Design review of the part built by this model. Coordinates are the model's own, in mm. A direction names the side the tool comes from. Coordinates: 2 decimals unless noted, no trailing zeros. Order: outer loops, then holes, each group sorted by start corner. A loop starts at its lowest first (then second) coordinate and runs counter-clockwise, first axis right, second up. Notation, with made-up numbers: M -24.75,9 L 13.25,9 A25 cw 13.25,41 Z; hole C 20,12.5 d3. An arc over 180 degrees is marked long. Answer in a Markdown table with one row per item.
Autodesk Inventor part; units mm, degrees
ref_plane "YZ Plane" through (0, 0, 0) normal (1, 0, 0) x (0, 1, 0)
ref_plane "XZ Plane" through (0, 0, 0) normal (0, 1, 0) x (-1, 0, 0)
ref_plane "XY Plane" through (0, 0, 0) normal (0, 0, 1) x (1, 0, 0)
sketch "Boceto16" plane through (0, 0, 0) normal (0, 0, 1) x (1, 0, 0)
  line L0 (-21.15, 21.15) -> (21.15, 21.15)
  line L1 (21.15, 21.15) -> (21.15, -21.15)
  line L2 (21.15, -21.15) -> (-21.15, -21.15)
  line L3 (-21.15, -21.15) -> (-21.15, 21.15)
  line L4 (2.3235, 0) -> (0, 0)
  line L5 (0, 0) -> (0, 2.4447)
  dimension "d75" = 42.3
  dimension "d76" = 42.3
extrude "Extrusión15" add sketch "Boceto16" along normal blind 15
sketch "Boceto17" plane through (0, 0, 15) normal (0, 0, 1) x (1, 0, 0)
  circle A0 centre (15.5, 15.5) radius 1.5
  point P0 (0, 0)
  dimension "d79" = 3
  dimension "d80" = 15.5
  dimension "d81" = 15.5
extrude "Extrusión16" cut sketch "Boceto17" against normal through all
pattern_linear "Patrón rectangular2" count 2 spacing 31 along (-1, 0, 0) count 2 spacing 31 along (0, -1, 0) of "Extrusión16"
sketch "Boceto18" plane through (0, 0, 15) normal (0, 0, 1) x (1, 0, 0)
  line L0 (-21.15, -21.15) -> (21.15, -21.15)
  line L1 (-21.15, 21.15) -> (-21.15, -21.15)
  line L2 (21.15, -21.15) -> (-21.15, -21.15)
  line L3 (-21.15, -21.15) -> (-21.15, 11.85)
  line L4 (-21.15, 11.85) -> (21.15, 11.85)
  line L5 (21.15, 11.85) -> (21.15, -21.15)
  circle A0 centre (-15.5, -15.5) radius 1.5
  circle A1 centre (15.5, -15.5) radius 1.5
  circle A2 centre (-15.5, 15.5) radius 1.5
  circle A3 centre (15.5, 15.5) radius 1.5
  line L6 (-21.15, -21.15) -> (21.15, -21.15)
  line L7 (21.15, -21.15) -> (21.15, 21.15)
  line L8 (21.15, 21.15) -> (-21.15, 21.15)
  line L9 (-21.15, 21.15) -> (-21.15, -21.15)
  point P0 (0, 0)
  point P1 (21.15, 11.85)
  dimension "d90" = 33
extrude "Extrusión17" cut sketch "Boceto18" against normal through all contours L1 L8 L7 L4
sketch "Boceto19" plane through (0, 0, 15) normal (0, 0, 1) x (1, 0, 0)
  circle A0 centre (0, 0) radius 11.25
  dimension "d93" = 22.5
extrude "Extrusión18" cut sketch "Boceto19" against normal through all
sketch "Boceto20" plane through (21.15, -21.15, 15) normal (1, 0, 0) x (0, 0, -1)
  line L0 (0, 0) -> (0, 33)
  circle A0 centre (0, 21.15) radius 1.5
  circle A1 centre (3, 21.15) radius 1.5
  line L1 (15, 33) -> (0, 33)
  line L2 (3, 22.65) -> (0, 22.65)
  line L3 (0, 19.65) -> (3, 19.65)
  line L4 (0, 9.9) -> (0, 32.4)
  line L5 (3, 21.15) -> (2.4132, 21.15)
  line L6 (15, 21.15) -> (14.0554, 21.15)
  dimension "d99" = 3
  dimension "d102" = 3
  dimension "d103" = 3
extrude "Extrusión19" cut sketch "Boceto20" against normal up to surface contours L0 A0 | A0 A1 L3 | L2 A1 A0 | A1 picked at (0.2169, 21.6005)
fillet "Empalme3" radius 1 2 edges at (16.1498, 1.5, 15) (16.1498, -1.5, 15)
sketch "Boceto21" plane through (-21.15, 11.85, 15) normal (0, 1, 0) x (1, 0, 0)
  circle A0 centre (32.3, 7.5) radius 2
  circle A1 centre (10.3, 7.5) radius 2
  line L0 (0, 15) -> (42.3, 15)
  line L1 (42.3, 15) -> (42.3, 0)
  line L2 (0, 0) -> (0, 15)
  point P0 (21.15, 15)
  dimension "d105" = 4
  dimension "d106" = 4
  dimension "d107" = 7.5
  dimension "d108" = 7.5
  dimension "d111" = 10
  dimension "d115" = 32
extrude "Extrusión20" cut sketch "Boceto21" against normal blind 5
equation "\"d102\" = d99"
equation "\"d106\" = d105"
equation "\"d107\" = d108"
properties part number "Soporte Motor Izq" material "Polietileno, baja densidad"
(1) Add section A-A, the plane y = -15.5. Give the boundary of the cut face in (x, z).
Return value:
| item | result |
|---|---|
| outline | M -21.15,0 L -17,0 L -17,15 L -21.15,15 Z; M -14,0 L 14,0 L 14,15 L -14,15 Z; M 17,0 L 21.15,0 L 21.15,15 L 17,15 Z |
(2) Insertion check: pin 1 Ø2.5 at (x, z) = (11.15, 7.5) entering from +Y; pin 2 Ø1.8 at (x, y) = (15.5, -15.5) entering from -Z. Each pin has a flat end and moves straight along its axis. Give the tip position at first contact, or say it passes through.
Return value:
| item | result |
|---|---|
| pin 1 | stops at y = 6.85 |
| pin 2 | passes through |
(3) Add section D-D, the plane x = 15.5. Give the boundary of the cut face in (y, z).
Return value:
| item | result |
|---|---|
| outline | M -21.15,0 L -17,0 L -17,15 L -21.15,15 Z; M -14,0 L 11.85,0 L 11.85,15 L 2.5,15 A1 ccw 1.5,14 L 1.5,12 A1.5 cw -1.5,12 L -1.5,14 A1 ccw -2.5,15 L -14,15 Z |
(4) Add section B-B, the plane x = 0. Give the boundary of the cut face in (y, z), and give its area (4 significant figures).
Return value:
| item | result |
|---|---|
| outline | M -21.15,0 L -11.25,0 L -11.25,15 L -21.15,15 Z; M 11.25,0 L 11.85,0 L 11.85,15 L 11.25,15 Z |
| area | 157.5 mm2 |
(5) For faces 5 (the flat face through (-11, 6.85, 7)), 6 (the cylindrical face through (16.2, 0, 10.5)), 7 (the cylindrical face through (14, -15.43, 7.6)), list the 3-axis set-ups (+Z, -Z, +X, -X, +Y, -Y) from which the entire face can be reached by the end or side of a thin tool; tool diameter is ignored.
Return value:
| item | result |
|---|---|
| face 5 | +Y |
| face 6 | +Z, +X |
| face 7 | +Z, -Z |
(6) Add section C-C, the plane z = 4.75. Give the boundary of the cut face in (x, y).
Return value:
| item | result |
|---|---|
| outline | M -21.15,-21.15 L 21.15,-21.15 L 21.15,11.85 L -21.15,11.85 Z; hole C -15.5,-15.5 d3; hole C 0,0 d22.5; hole C 15.5,-15.5 d3 |
(7) Draft analysis for pull direction X (two halves, no side actions). For faces 1 (the flat face through (11, 6.85, 7)), 2 (the flat face through (21.15, -4, 7)), 3 (the flat face through (16, 1.5, 13)), 4 (the cylindrical face through (-8.942, 9.385, 6.899)), state which applies: pulls with the +X half, pulls with the -X half, needs draft (parallel to the pull), parting line crosses it, or undercut.
Return value:
| item | result |
|---|---|
| face 1 | undercut |
| face 2 | pulls with the +X half |
| face 3 | needs draft |
| face 4 | undercut |
(8) For line 1 along Y through (x, z) = (19, 12.75); line 2 along X through (y, z) = (0, 8.5); line 3 along Y through (x, z) = (15.5, 9.5), list the stretches that pass through material, from the lowest coordinate up. Write a range as from..to.
Return value:
| item | result |
|---|---|
| line 1 | y = -21.15..-1.5, 1.5..11.85 |
| line 2 | x = -21.15..-11.25, 11.25..21.15 |
| line 3 | y = -21.15..-17, -14..11.85 |
